Read the model definition and answer for the solid it produces. Units are mm, in the model's axes. Coordinates: 2 decimals unless noted, no trailing zeros. Loops run counter-clockwise (first coordinate to the right, second up) from the corner with the lowest first, then second, coordinate; pieces in that order, holes last.
from build123d import *

# Parameters (mm, degrees)
SKETCH1_W          = 130
SKETCH1_H          = 70
BASE_FLANGE1_DEPTH = 3
SKETCH12_R         = 2.5
SKETCH12_R_2       = 2
CUT_EXTRUDE1_DEPTH = 10
SKETCH13_R         = 3.75
CUT_EXTRUDE2_DEPTH = 10


# Sheet-metal steps are written as plain solids
with BuildPart() as part:
    # Sketch1 → Base-Flange1 (new body)
    with BuildSketch(Plane.XY):
        Rectangle(SKETCH1_W, SKETCH1_H)
    extrude(amount=BASE_FLANGE1_DEPTH)

    # Sketch12 → Cut-Extrude1 (cut)
    with BuildSketch(Plane(origin=(0, 0, 0), x_dir=(-1, 0, 0), z_dir=(0, 0, -1))):
        with Locations((56, 16)):
            Circle(SKETCH12_R)
        with Locations((56, -16)):
            Circle(SKETCH12_R)
        with Locations((24, -16)):
            Circle(SKETCH12_R)
        with Locations((24, 16)):
            Circle(SKETCH12_R)
        with Locations(Location((-24, 16, 0), (0, 0, 180))):
            Circle(SKETCH12_R)
        with Locations(Location((-24, -16, 0), (0, 0, 180))):
            Circle(SKETCH12_R)
        with Locations(Location((-56, -16, 0), (0, 0, 180))):
            Circle(SKETCH12_R)
        with Locations(Location((-56, 16, 0), (0, 0, 180))):
            Circle(SKETCH12_R)
        with Locations((12, 9)):
            Circle(SKETCH12_R_2)
        with Locations(Location((-12, 9, 0), (0, 0, 180))):
            Circle(SKETCH12_R_2)
        with Locations((-12, -9)):
            Circle(SKETCH12_R_2)
        with Locations(Location((12, -9, 0), (0, 0, 180))):
            Circle(SKETCH12_R_2)
    extrude(amount=-CUT_EXTRUDE1_DEPTH, mode=Mode.SUBTRACT)

    # Sketch13 → Cut-Extrude2 (cut)
    with BuildSketch(Plane(origin=(0, 0, 0), x_dir=(-1, 0, 0), z_dir=(0, 0, -1))):
        with Locations((35, 10)):
            Circle(SKETCH13_R)
        with Locations((-35, 10)):
            Circle(SKETCH13_R)
        with Locations((-35, -10)):
            Circle(SKETCH13_R)
        with Locations((35, -10)):
            Circle(SKETCH13_R)
    extrude(amount=-CUT_EXTRUDE2_DEPTH, mode=Mode.SUBTRACT)


solid = part.part
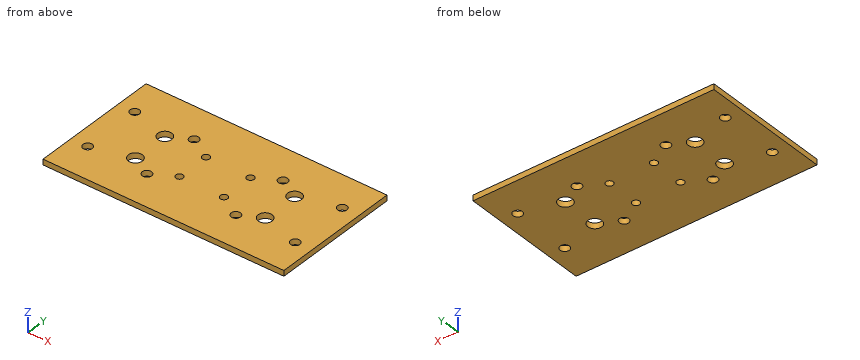
Q1. A cutting plane is placed at A-A (x = 56). Give the vertices of the cut face in (y, z), then the cut area to 3 significant figures.
Findings below:
outline: (-35, 0) - (-18.5, 0) - (-18.5, 3) - (-35, 3) - close; (-13.5, 0) - (13.5, 0) - (13.5, 3) - (-13.5, 3) - close; (18.5, 0) - (35, 0) - (35, 3) - (18.5, 3) - close
area: 180 mm2
Q2. Straight lines are drawn through the part: probe 1 along Y at (x, z) = (-24, 0.75); probe 2 along Y at (x, z) = (-35, 1.75); probe 3 along X at (y, z) = (-8, 1.15). For each, find the intervals that lie inside material, in ascending order.
Findings below:
probe 1: y = -35 to -18.5, -13.5 to 13.5, 18.5 to 35
probe 2: y = -35 to -13.75, -6.25 to 6.25, 13.75 to 35
probe 3: x = -65 to -38.17, -31.83 to -13.73, -10.27 to 10.27, 13.73 to 31.83, 38.17 to 65
Q3. A cutting plane is placed at C-C (x = 12). Give the vertices of the cut face in (y, z), then the cut area to 3 significant figures.
Findings below:
outline: (-35, 0) - (-11, 0) - (-11, 3) - (-35, 3) - close; (-7, 0) - (7, 0) - (7, 3) - (-7, 3) - close; (11, 0) - (35, 0) - (35, 3) - (11, 3) - close
area: 186 mm2
Q4. A cutting plane is placed at B-B (z = 0.65). Count the separate pieces of the cut face and the enclosed holes in it, then the cut area to 3 significant figures.
Findings below:
separate pieces: 1
enclosed holes: 16
area: 8,720 mm2
